Input: part model. Units: mm. Frame: model coordinates. Face numbers are marked on the shaded views. Round coordinates to 2 decimals unless told otherwise and drop trailing zeros. Write each loop counter-clockwise with the first axis right and the second up, starting at its lowest first coordinate (ties: lowest second). Pieces come first, ordered by that corner, then holes. Notation, with made-up numbers: (88.5, 78) - (126.5, 78) arc R13 cw to (126.5, 82) - close; hole circle Ø10 at (80, -39.5). An arc over 180 degrees is marked (long way). One line per item, written item: value. Start each with the question number.
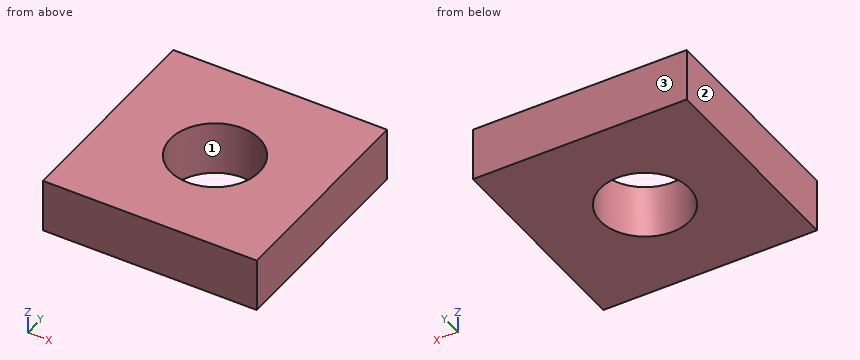
```python
from build123d import *

# Parameters (mm, degrees)
PLAT_W                      = 60
PLAT_H                      = 15
EL_MENT_M_CANO_SOUD_1_DEPTH = 60
ESQUISSE2_R                 = 12.5
ENL_V_MAT_EXTRU_1_DEPTH     = 20


with BuildPart() as part:
    # plat → Elément mécano-soudé1 (new body)
    with BuildSketch(Plane.YZ.offset(-30)):
        Rectangle(PLAT_W, PLAT_H)
    extrude(amount=EL_MENT_M_CANO_SOUD_1_DEPTH)

    # Esquisse2 → Enlèv. mat.-Extru.1 (cut)
    with BuildSketch(Plane.XY.offset(7.5)):
        Circle(ESQUISSE2_R)
    extrude(amount=-ENL_V_MAT_EXTRU_1_DEPTH, mode=Mode.SUBTRACT)


solid = part.part
```
Q1. Contact query for a flat-ended pin moving along its axis: pin 1 Ø22.5 at (x, y) = (0, 0) entering from +Z. Output: stop coordinate, or through.
Q2. Cut plane B-B, the plane y = 0. Output: boundary loops of the cut face in (x, z), and give its area (3 significant figures).
Q3. Cut plane A-A, the plane x = -7.5. Output: boundary loops of the cut face in (y, z).
Q4. Pull-direction query (Y, two-part tool) for the marked faces 1, 2 and 3; classes: pulls with the +Y half, pulls with the -Y half, needs draft (parallel to the pull), parting line crosses it, or undercut.
Q5. Material intervals for probe 1 along Y at (x, z) = (0, 2.5); probe 2 along Y at (x, z) = (10.5, 1.25); probe 3 along X at (y, z) = (-8, -6), sorted ascending. Write a range as from..to.
Q6. Cut plane C-C, the plane z = 2.75. Output: boundary loops of the cut face in (x, y).
A:
1. pin 1: passes through
2. outline: (-30, -7.5) - (-12.5, -7.5) - (-12.5, 7.5) - (-30, 7.5) - close; (12.5, -7.5) - (30, -7.5) - (30, 7.5) - (12.5, 7.5) - close
2. area: 525 mm²
3. outline: (-30, -7.5) - (-10, -7.5) - (-10, 7.5) - (-30, 7.5) - close; (10, -7.5) - (30, -7.5) - (30, 7.5) - (10, 7.5) - close
4. face 1: undercut
4. face 2: needs draft
4. face 3: pulls with the +Y half
5. probe 1: y = -30..-12.5, 12.5..30
5. probe 2: y = -30..-6.78, 6.78..30
5. probe 3: x = -30..-9.6, 9.6..30
6. outline: (-30, -30) - (30, -30) - (30, 30) - (-30, 30) - close; hole circle Ø25 at (0, 0)
